```python
from build123d import *

# Parameters (mm, degrees)
SKETCH_R        = 1.55
SKETCH_R_2      = 1.5
SKETCH_R_3      = 3.65
SKETCH_R_4      = 1.4
SKETCH_W        = 8
SKETCH_H        = 3
SKETCH_W_2      = 12.7
PAD_DEPTH       = 9.5
POCKET_DEPTH    = 7
POCKET001_DEPTH = 10
POCKET002_DEPTH = 4.5
POCKET003_DEPTH = 4.5
SKETCH005_W     = 25.7
SKETCH005_H     = 13
POCKET004_DEPTH = 3
POCKET006_DEPTH = 2.5
SKETCH006_R     = 1.8
POCKET007_DEPTH = 1.5
FILLET_R        = 1
FILLET001_R     = 0.5
POCKET008_DEPTH = 2.2


with BuildPart() as part:
    # Sketch → Pad (new body)
    with BuildSketch(Plane.XY):
        with BuildLine():
            Line((-11, 13.5), (7.5, 13.5))
            ThreePointArc((15.5, 5.5), (13.156854, 11.156854), (7.5, 13.5))
            Line((15.5, 5.5), (15.5, -25.53))
            ThreePointArc((12.7, -28.33), (14.679899, -27.509899), (15.5, -25.53))
            Line((11, -28.33), (12.7, -28.33))
            Line((11, -29.53), (11, -28.33))
            Line((-3, -29.53), (11, -29.53))
            Line((-3, -31.13), (-3, -29.53))
            Line((-3, -31.13), (-16, -31.13))
            Line((-16, -31.13), (-16, 8.5))
            ThreePointArc((-11, 13.5), (-14.535534, 12.035534), (-16, 8.5))
        make_face()
        with Locations((-11, -11)):
            Circle(SKETCH_R, mode=Mode.SUBTRACT)
        with Locations((11, -11)):
            Circle(SKETCH_R, mode=Mode.SUBTRACT)
        with Locations((8.5, 8.5)):
            Circle(SKETCH_R_2, mode=Mode.SUBTRACT)
        with Locations((-10.5, 7)):
            Circle(SKETCH_R_2, mode=Mode.SUBTRACT)
        with Locations((0.5, 0)):
            Circle(SKETCH_R_3, mode=Mode.SUBTRACT)
        with Locations((-5.5, 8.5)):
            Circle(SKETCH_R_4, mode=Mode.SUBTRACT)
        with Locations((-8.7, -25.79)):
            Rectangle(SKETCH_W, SKETCH_H, mode=Mode.SUBTRACT)
        with Locations((6.35, -25.79)):
            Rectangle(SKETCH_W_2, SKETCH_H, mode=Mode.SUBTRACT)
    extrude(amount=PAD_DEPTH)

    # Sketch002 (on Face27 of Pad) → Pocket (cut)
    with BuildSketch(Plane.XY.offset(9.5)):
        with BuildLine():
            Line((7.85, -4), (7.75, -4))
            ThreePointArc((7.75, -4), (7.042893, -4.292893), (6.75, -5))
            Line((6.75, -5), (6.75, -5.35))
            ThreePointArc((5.85, -6.25), (6.486396, -5.986396), (6.75, -5.35))
            Line((5.85, -6.25), (-4.85, -6.25))
            ThreePointArc((-5.75, -5.35), (-5.486396, -5.986396), (-4.85, -6.25))
            Line((-5.75, -5.35), (-5.75, -5))
            ThreePointArc((-5.75, -5), (-6.042893, -4.292893), (-6.75, -4))
            Line((-6.75, -4), (-6.85, -4))
            ThreePointArc((-7.75, -3.1), (-7.486396, -3.736396), (-6.85, -4))
            Line((-7.75, -3.1), (-7.75, 3.1))
            ThreePointArc((-6.85, 4), (-7.486396, 3.736396), (-7.75, 3.1))
            Line((-6.85, 4), (-6.75, 4))
            ThreePointArc((-6.75, 4), (-6.042893, 4.292893), (-5.75, 5))
            Line((-5.75, 5), (-5.75, 5.35))
            ThreePointArc((-4.85, 6.25), (-5.486396, 5.986396), (-5.75, 5.35))
            Line((-4.85, 6.25), (5.85, 6.25))
            ThreePointArc((6.75, 5.35), (6.486396, 5.986396), (5.85, 6.25))
            Line((6.75, 5.35), (6.75, 5))
            ThreePointArc((6.75, 5), (7.042893, 4.292893), (7.75, 4))
            Line((7.75, 4), (7.85, 4))
            ThreePointArc((8.75, 3.1), (8.486396, 3.736396), (7.85, 4))
            Line((8.75, 3.1), (8.75, -3.1))
            ThreePointArc((7.85, -4), (8.486396, -3.736396), (8.75, -3.1))
        make_face()
    extrude(amount=-POCKET_DEPTH, mode=Mode.SUBTRACT)

    # Sketch007 (on Face5 of Pocket) → Pocket001 (cut)
    with BuildSketch(Plane.XY.offset(9.5)):
        with BuildLine():
            Line((12.75, 7), (16.5, 7))
            Line((16.5, 7), (16.5, -7))
            Line((16.5, -7), (12.75, -7))
            ThreePointArc((11.5, -5.75), (11.866117, -6.633883), (12.75, -7))
            Line((11.5, -5.75), (11.5, 5.75))
            ThreePointArc((12.75, 7), (11.866117, 6.633883), (11.5, 5.75))
        make_face()
    extrude(amount=-POCKET001_DEPTH, mode=Mode.SUBTRACT)

    # Sketch008 (on Face5 of Pocket001) → Pocket002 (cut)
    with BuildSketch(Plane.XY.offset(9.5)):
        Polygon((-8.1, -12.674316), (-8.1, -9.325684), (-11, -7.651368), (-13.9, -9.325684), (-13.9, -12.674316), (-11, -14.348632), align=None)
        Polygon((13.9, -12.674316), (13.9, -9.325684), (11, -7.651368), (8.1, -9.325684), (8.1, -12.674316), (11, -14.348632), align=None)
    extrude(amount=-POCKET002_DEPTH, mode=Mode.SUBTRACT)

    # Sketch009 (on Face5 of Pocket002) → Pocket003 (cut)
    with BuildSketch(Plane.XY.offset(9.5)):
        Polygon((-7.85, 5.470022), (-7.85, 8.529978), (-10.5, 10.059956), (-13.15, 8.529978), (-13.15, 5.470022), (-10.5, 3.940044), align=None)
    extrude(amount=-POCKET003_DEPTH, mode=Mode.SUBTRACT)

    # Sketch005 (on Face4 of Pocket003) → Pocket004 (cut)
    with BuildSketch(Plane(origin=(0, 0, 0), x_dir=(1, 0, 0), z_dir=(0, 0, -1))):
        with Locations((0, 22)):
            Rectangle(SKETCH005_W, SKETCH005_H)
    extrude(amount=-POCKET004_DEPTH, mode=Mode.SUBTRACT)

    # Sketch010 → Pocket006 (cut)
    with BuildSketch(Plane(origin=(0, 0, 0), x_dir=(1, 0, 0), z_dir=(0, 0, -1))):
        with BuildLine():
            Line((-16, -10), (-11, -10))
            ThreePointArc((-10, -11), (-10.292893, -10.292893), (-11, -10))
            Line((-10, -11), (-10, -14))
            Line((-10, -14), (-16, -14))
            Line((-16, -14), (-16, -10))
        make_face()
    extrude(amount=-POCKET006_DEPTH, mode=Mode.SUBTRACT)

    # Sketch006 (on Face83 of Pocket006) → Pocket007 (cut)
    with BuildSketch(Plane(origin=(0, 0, 3), x_dir=(1, 0, 0), z_dir=(0, 0, -1))):
        with Locations((0, 22)):
            Circle(SKETCH006_R)
        with BuildLine():
            Line((-12.85, 20.5), (-3.5, 20.5))
            ThreePointArc((-1.5, 18.5), (-2.085786, 19.914214), (-3.5, 20.5))
            Line((-1.5, 18.5), (-1.5, 15.5))
            Line((-1.5, 15.5), (-12.85, 15.5))
            Line((-12.85, 15.5), (-12.85, 20.5))
        make_face()
        with BuildLine():
            Line((1.5, 15.5), (12.85, 15.5))
            Line((12.85, 15.5), (12.85, 20.5))
            Line((12.85, 20.5), (3.5, 20.5))
            ThreePointArc((3.5, 20.5), (2.085786, 19.914214), (1.5, 18.5))
            Line((1.5, 18.5), (1.5, 15.5))
        make_face()
        with BuildLine():
            Line((-12.85, 23.5), (-3.5, 23.5))
            ThreePointArc((-3.5, 23.5), (-2.085786, 24.085786), (-1.5, 25.5))
            Line((-1.5, 25.5), (-1.5, 28.5))
            Line((-1.5, 28.5), (-12.85, 28.5))
            Line((-12.85, 28.5), (-12.85, 23.5))
        make_face()
        with BuildLine():
            Line((1.5, 28.5), (12.85, 28.5))
            Line((12.85, 28.5), (12.85, 23.5))
            Line((12.85, 23.5), (3.5, 23.5))
            ThreePointArc((1.5, 25.5), (2.085786, 24.085786), (3.5, 23.5))
            Line((1.5, 25.5), (1.5, 28.5))
        make_face()
    extrude(amount=-POCKET007_DEPTH, mode=Mode.SUBTRACT)

    # Fillet
    fillet_edges = [part.edges().sort_by_distance(p)[0] for p in [
        (15.358117, 7, 4.75),
        (15.5, -7, 4.75),
        (11, -29.53, 4.75),
        (-3, -31.13, 4.75),
        (-16, -31.13, 4.75),
        (-15.769696, 10, 1.25),
        (-10, 13.5, 1.25),
    ]]
    fillet(fillet_edges, radius=FILLET_R)

    # Fillet001
    fillet001_edges = [part.edges().sort_by_distance(p)[0] for p in [
        (-3, -29.53, 4.75),
        (-12.85, -15.5, 1.5),
        (-12.85, -15.5, 3.75),
        (1.5, -15.5, 3.75),
        (-12.85, -23.5, 3.75),
        (-12.85, -28.5, 3.75),
        (-12.85, -28.5, 1.5),
        (-12.85, -20.5, 3.75),
        (-12.7, -27.29, 7),
        (-1.5, -15.5, 3.75),
        (-4.7, -24.29, 7),
        (-4.7, -27.29, 7),
        (-12.7, -24.29, 7),
        (-1.5, -28.5, 3.75),
        (1.5, -28.5, 3.75),
        (1.5, -27.29, 3.75),
        (0, -27.29, 6.25),
        (0, -24.29, 6.25),
        (1.907549, -24.29, 3.75),
        (12.85, -20.5, 3.75),
        (12.7, -27.29, 7),
        (12.85, -23.5, 3.75),
        (12.85, -15.5, 3.75),
        (12.85, -15.5, 1.5),
        (12.7, -24.29, 7),
        (-1.8, -22, 4.5),
    ]]
    fillet(fillet001_edges, radius=FILLET001_R)

    # Sketch011 (on Face1 of Fillet001) → Pocket008 (cut)
    with BuildSketch(Plane(origin=(0, 0, 0), x_dir=(1, 0, 0), z_dir=(0, 0, -1))):
        Polygon((-2.85, -10.029978), (-2.85, -6.970022), (-5.5, -5.440044), (-8.15, -6.970022), (-8.15, -10.029978), (-5.5, -11.559956), align=None)
    extrude(amount=-POCKET008_DEPTH, mode=Mode.SUBTRACT)


solid = part.part
```
The listing builds one solid part. Answer for the finished solid, in the listing's coordinates (mm). A direction names the side the tool comes from. Give positions to 0.01 mm unless a question says otherwise; leave off trailing zeros. Write each loop counter-clockwise with the first axis right and the second up, starting at its lowest first coordinate (ties: lowest second). Pieces come first, ordered by that corner, then holes. Notation, with made-up numbers: (-17, 0) - (32, 0) arc R19 cw to (32, 26) - close; hole circle Ø5 at (-31.5, 63.25). An arc over 180 degrees is marked (long way). Use one line per item in the form item = value. Start each with the question number.
1) A tool of negligible diameter and unlimited length cuts with its end or side. For faces 1 (the face through (11.856, -6.624, 4.816)), 2 (the face through (-7.85, 7, 7)), 3 (the face through (-0.234, -23.785, 3.493)), 4 (the face through (0, -26, 6)), from which of +Z, -Z, +X, -X, +Y, -Y can it reach the whole face along a straight path? Write none if from no direction.
2) The mould has two halves that part along X. Classify faces 5 (the face through (15.215, -7.301, 4.816)), 6 (the face through (9.53, -13.5, 7.28)), 7 (the face through (-12, 12, 2.5)): pulls with the +X half, pulls with the -X half, needs draft (parallel to the pull), parting line crosses it, or undercut.
3) Find section A-A on y = -11. Determine the outline of the cut face in (x, z).
4) Consider line 1 along Y through (x, z) = (5, 6.75); line 2 along X through (y, z) = (-20, 0.75); line 3 along Y through (x, z) = (13, 6). Determine where each line is inside the solid, lowest interval first. Write a range as from..to.
5) Find section C-C on z = 1.5. Count the separate pieces of the cut face and the enclosed holes in it, plus the area to 3 significant figures.
6) Find section B-B on y = 0. Determine the outline of the cut face in (x, z), plus the area to 4 significant figures.
7) Flat-ended cylindrical pins translate along their axes: pin 1 Ø0.8 at (x, z) = (12, 6.5) entering from -Y; pin 2 Ø1 at (x, y) = (8.5, -25.5) entering from -Z; pin 3 Ø1.5 at (x, z) = (-0.5, 3.5) entering from -Y. Find the tip coordinate at first contact, or state that the pin passes through.
Geometry results:
q1.face_1 = +Z, -Z, +X
q1.face_2 = +Z
q1.face_3 = -Z
q1.face_4 = +Z, -Z
q2.face_5 = pulls with the +X half
q2.face_6 = undercut
q2.face_7 = needs draft
q3.outline = (-16, 0) - (-12.55, 0) - (-12.55, 5) - (-13.9, 5) - (-13.9, 9.5) - (-16, 9.5) - close; (-9.45, 0) - (9.45, 0) - (9.45, 5) - (8.1, 5) - (8.1, 9.5) - (-8.1, 9.5) - (-8.1, 5) - (-9.45, 5) - close; (12.55, 0) - (15.5, 0) - (15.5, 9.5) - (13.9, 9.5) - (13.9, 5) - (12.55, 5) - close
q4.line_1 = -29.53..-27.29, -24.29..-6.25, 6.25..13.5
q4.line_2 = -16..-12.85, 12.85..15.5
q4.line_3 = -28.31..-13.19, -8.81..-7, 7..11.31
q5.separate_pieces = 1
q5.enclosed_holes = 6
q5.area = 849 mm2
q6.outline = (-16, 0) - (-3.15, 0) - (-3.15, 2.5) - (-7.75, 2.5) - (-7.75, 9.5) - (-16, 9.5) - close; (4.15, 0) - (11.5, 0) - (11.5, 9.5) - (8.75, 9.5) - (8.75, 2.5) - (4.15, 2.5) - close
q6.area = 127.5 mm2
q7.pin_1 = -28.33
q7.pin_2 = through
q7.pin_3 = -29.53
